from build123d import *

# Parameters (mm, degrees)
SKETCH1_R           = 42.5
BOSS_EXTRUDE1_DEPTH = 102.5
SKETCH2_R           = 90
SKETCH2_R_2         = 42.5
BOSS_EXTRUDE2_DEPTH = 5
SKETCH3_R           = 90
SKETCH3_R_2         = 42.5
BOSS_EXTRUDE3_DEPTH = 5
BOSS_EXTRUDE4_DEPTH = 75
BOSS_EXTRUDE5_DEPTH = 75
FILLET2_R           = 15
SKETCH6_R           = 42.5
BOSS_EXTRUDE6_DEPTH = 205


with BuildPart() as part:
    # Sketch1 → Boss-Extrude1 (new body, symmetric)
    with BuildSketch(Plane.XY):
        with BuildLine():
            ThreePointArc((-52.068634079, 99.725159038), (-72.31360609, -86.179999851), (107.251733212, -33.960502395))
            ThreePointArc((107.251733212, -33.960502395), (160.82695798, 70.255427056), (245.798784868, 150.946525051))
            ThreePointArc((245.798784868, 150.946525051), (253.901105826, 302.587555032), (105.970797095, 268.276138019))
            ThreePointArc((105.970797095, 268.276138019), (41.260781083, 170.583361992), (-52.068634079, 99.725159038))
        make_face()
        Circle(SKETCH1_R, mode=Mode.SUBTRACT)
    extrude(amount=BOSS_EXTRUDE1_DEPTH, both=True)

    # Sketch2 → Boss-Extrude2 (add)
    with BuildSketch(Plane.XY.offset(102.5)):
        Circle(SKETCH2_R)
        Circle(SKETCH2_R_2, mode=Mode.SUBTRACT)
    extrude(amount=BOSS_EXTRUDE2_DEPTH)

    # Sketch3 → Boss-Extrude3 (add)
    with BuildSketch(Plane(origin=(0, 0, -102.5), x_dir=(-1, 0, 0), z_dir=(0, 0, -1))):
        Circle(SKETCH3_R)
        Circle(SKETCH3_R_2, mode=Mode.SUBTRACT)
    extrude(amount=BOSS_EXTRUDE3_DEPTH)

    # Sketch4 → Boss-Extrude4 (add)
    with BuildSketch(Plane.XY.offset(102.5)):
        with BuildLine():
            ThreePointArc((339.810505034, 840.887250831), (167.534603821, 563.507294819), (69.811758527, 251.948517629))
            ThreePointArc((69.811758527, 251.948517629), (180.075530777, 105.466386029), (317.792368114, 226.500212138))
            ThreePointArc((317.792368114, 226.500212138), (358.459856731, 500.613644392), (463.518163787, 757.040574513))
            ThreePointArc((463.518163787, 757.040574513), (440.127359965, 855.712385585), (339.810505034, 840.887250831))
        make_face()
    extrude(amount=BOSS_EXTRUDE4_DEPTH)

    # Sketch5 → Boss-Extrude5 (add)
    with BuildSketch(Plane(origin=(0, 0, -102.5), x_dir=(-1, 0, 0), z_dir=(0, 0, -1))):
        with BuildLine():
            ThreePointArc((-317.792368114, 226.500212138), (-180.075530777, 105.466386029), (-69.811758527, 251.948517629))
            ThreePointArc((-69.811758527, 251.948517629), (-167.534603821, 563.507294819), (-339.810505034, 840.887250831))
            ThreePointArc((-339.810505034, 840.887250831), (-440.127359965, 855.712385585), (-463.518163787, 757.040574513))
            ThreePointArc((-463.518163787, 757.040574513), (-358.459856731, 500.613644392), (-317.792368114, 226.500212138))
        make_face()
    extrude(amount=BOSS_EXTRUDE5_DEPTH)

    # Fillet2
    fillet2_edges = [part.edges().sort_by_distance(p)[0] for p in [
        (167.534603821, 563.507294819, 177.5),
        (180.075530777, 105.466386029, 177.5),
        (358.459856731, 500.613644392, 177.5),
        (440.127359965, 855.712385585, 177.5),
        (358.459856731, 500.613644392, -177.5),
        (180.075530777, 105.466386029, -177.5),
        (167.534603821, 563.507294819, -177.5),
        (440.127359965, 855.712385585, -177.5),
    ]]
    fillet(fillet2_edges, radius=FILLET2_R)

    # Sketch6 → Boss-Extrude6 (add)
    with BuildSketch(Plane.XY.offset(-102.5)):
        with Locations((398.048368901, 793.628905407)):
            Circle(SKETCH6_R)
        with BuildLine():
            ThreePointArc((419.855651368, 670.545834145), (361.07481022, 509.978649739), (326.751661219, 342.470651611))
            ThreePointArc((326.751661219, 342.470651611), (219.389147641, 402.787161518), (98.878270441, 377.451037787))
            ThreePointArc((98.878270441, 377.451037787), (172.976016961, 575.222465787), (278.119497696, 758.385950771))
            ThreePointArc((278.119497696, 758.385950771), (332.200566612, 687.378884543), (419.855651368, 670.545834145))
        make_face()
    extrude(amount=BOSS_EXTRUDE6_DEPTH)


solid = part.part
Work out the finished part from the listing and answer in its coordinate system (mm). A direction names the side the tool comes from. Coordinates: 2 decimals unless noted, no trailing zeros. Write each loop counter-clockwise with the first axis right and the second up, starting at its lowest first coordinate (ties: lowest second). Pieces come first, ordered by that corner, then holes.
1. The part is cut by section A-A, the plane z = 14. Write down the section's boundary in (x, y), and give its area (3 significant figures).
Results list:
outline: (-52.07, 99.73) arc R112.5 ccw (long way) to (107.25, -33.96) arc R350 cw to (245.8, 150.95) arc R95 ccw (long way) to (105.97, 268.28) arc R350 cw to start; (98.88, 377.45) arc R175 cw to (326.75, 342.47) arc R1150 cw to (419.86, 670.55) arc R125 cw to (278.12, 758.39) arc R1300 ccw to start; circle Ø85 at (398.05, 793.63); hole circle Ø85 at (0, 0)
area: 153,000 mm2
2. Consider line 1 along Z through (x, y) = (164.5, 379.5); line 2 along Y through (x, z) = (0, -104); line 3 along X through (y, z) = (794, -51.5). Determine where each line is inside the solid, lowest interval first.
Results list:
line 1: z = -177.5 to -102.5, 102.5 to 177.5
line 2: y = -90 to -42.5, 42.5 to 90
line 3: x = 355.55 to 440.55
3. For a pull along Z with two mould halves and no side action, classify faces 5 (the flat face through (268, 492, 177.5)), 6 (the cylindrical face through (438.83, 856.57, -132.08)), 7 (the flat face through (224, 324, 102.5)) as +Z half, -Z half, draft (parallel to the pull), parting line (faces both ways), or undercut.
Results list:
face 5: +Z half
face 6: draft
face 7: undercut
4. The part is cut by section B-B, the plane x = 30.5. Write down the section's boundary in (y, z), and give its area (3 significant figures).
Results list:
outline: (-108.29, -102.5) - (-84.67, -102.5) - (-84.67, -107.5) - (-29.6, -107.5) - (-29.6, 107.5) - (-84.67, 107.5) - (-84.67, 102.5) - (-108.29, 102.5) - close; (29.6, -107.5) - (84.67, -107.5) - (84.67, -102.5) - (159.6, -102.5) - (159.6, 102.5) - (84.67, 102.5) - (84.67, 107.5) - (29.6, 107.5) - close
area: 43,900 mm2
5. The part is cut by section C-C, the plane y = 0. Write down the section's boundary in (x, z).
Results list:
outline: (-112.5, -102.5) - (-90, -102.5) - (-90, -107.5) - (-42.5, -107.5) - (-42.5, 107.5) - (-90, 107.5) - (-90, 102.5) - (-112.5, 102.5) - close; (42.5, -107.5) - (90, -107.5) - (90, -102.5) - (119.98, -102.5) - (119.98, 102.5) - (90, 102.5) - (90, 107.5) - (42.5, 107.5) - close
6. Flat-ended cylindrical pins translate along their axes: pin 1 (10 mm diameter, centred on x = 261.5, z = -112.5, fed in from +Y); pin 2 (3 mm diameter, centred on x = 175.5, z = 78.5, fed in from -Y); pin 3 (8 mm diameter, centred on x = 25, z = -28.5, fed in from -Y). Find the tip coordinate at first contact, or state that the pin passes through.
Results list:
pin 1: stops at y = 741.2
pin 2: stops at y = 86.77
pin 3: stops at y = -110.52
7. The part is cut by section D-D, the plane z = -124. Write down the section's boundary in (x, y).
Results list:
outline: (69.81, 251.95) arc R125 ccw (long way) to (317.79, 226.5) arc R1150 cw to (463.52, 757.04) arc R75 ccw to (339.81, 840.89) arc R1300 ccw to start
8. For faces 1 (the flat face through (228, 324, -102.5)), 2 (the cylindrical face through (-41.53, -79.845, -104.965)), 3 (the cylindrical face through (41.53, -79.845, 104.965)), 4 (the cylindrical face through (159.84, 68.93, 1.44)), determine the directions among +Z, -Z, +X, -X, +Y, -Y from which every point of the face is accessible in a straight line to the end or side of a thin tool.
Results list:
face 1: none
face 2: -Z
face 3: +Z
face 4: +X, -Y
